Part model, mm, in its own coordinate system. Face numbers are marked on the shaded views. A direction names the side the tool comes from. Round coordinates to 2 decimals unless told otherwise and drop trailing zeros. Order: outer loops, then holes, each group sorted by start corner. A loop starts at its lowest first (then second) coordinate and runs counter-clockwise, first axis right, second up. Notation, with made-up numbers: M 17.5,37 L 33.5,37 A16 ccw 33.5,42 Z; hole C 76.25,-1.75 d3. An arc over 180 degrees is marked long. One line per question, with ' | ' between items.
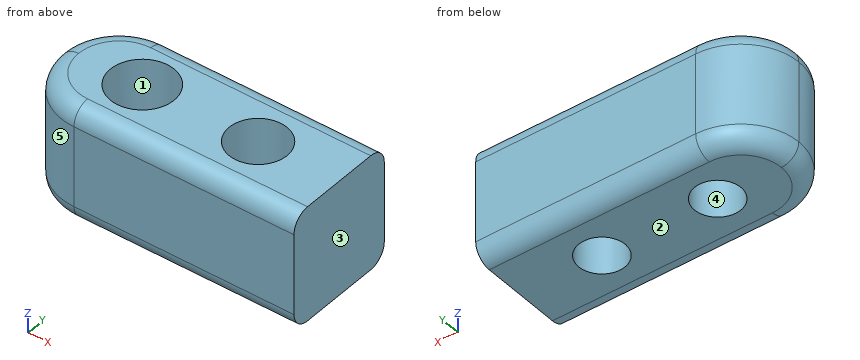
Autodesk Inventor part; units mm, degrees
ref_plane "YZ Plane" through (0, 0, 0) normal (1, 0, 0) x (0, 1, 0)
ref_plane "XZ Plane" through (0, 0, 0) normal (0, 1, 0) x (-1, 0, 0)
ref_plane "XY Plane" through (0, 0, 0) normal (0, 0, 1) x (1, 0, 0)
sketch "Sketch8" plane through (0, 0, 0) normal (0, 0, 1) x (1, 0, 0)
  line L0 (0, 0) -> (-10, 0)
  line L1 (-10, 0) -> (-10, 10)
  line L2 (-10, 10) -> (0, 10)
  line L3 (0, 10) -> (0, 0)
  dimension "d38" = 10
  dimension "d39" = 10
extrude "Extrusion5" add sketch "Sketch8" along normal blind 10
sketch "Sketch9" plane through (0, 0, 10) normal (0, 0, 1) x (1, 0, 0)
  point P0 (0, 0)
  point P1 (-5, 5)
hole "Hole3" at (-5, 5, 10) direction (0, 0, -1) diameter 4 depth 10 counterbore diameter 5.5 counterbore depth 5
sketch "Sketch14" plane through (-10, 0, 0) normal (-1, 0, 0) x (0, 0, 1)
  line L0 (0, 0) -> (10, 0)
  line L1 (10, 0) -> (10, 10)
  line L2 (10, 10) -> (0, 10)
  line L3 (0, 10) -> (0, 0)
  dimension "d71" = 10
  dimension "d72" = 10
extrude "Extrusion9" add sketch "Sketch14" along normal blind 2
fillet "Fillet1" radius 5 2 edges at (-12, 10, 5) (-12, 0, 5)
sketch "Sketch15" plane through (0, 0, 0) normal (1, 0, 0) x (0, 0, -1)
  line L0 (-10, 0) -> (-10, 10)
  line L1 (0, 0) -> (-10, 0)
  line L2 (-10, 0) -> (-10, 10)
  line L3 (-10, 10) -> (0, 10)
  line L4 (0, 10) -> (0, 0)
  dimension "d76" = 10
  dimension "d77" = 10
extrude "Extrusion10" add sketch "Sketch15" along normal blind 10
sketch "Sketch16" plane through (0, 0, 10) normal (0, 0, 1) x (1, 0, 0)
  point P0 (0, 0)
  point P1 (5, 5)
hole "Hole5" at (5, 5, 10) direction (0, 0, -1) diameter 4 depth 10 counterbore diameter 5 counterbore depth 4.5
sketch "Sketch17" plane through (10, 0, 0) normal (1, 0, 0) x (0, 0, -1)
  line L0 (0, 0) -> (-10, 0)
  line L1 (-10, 0) -> (-10, 10)
  line L2 (-10, 10) -> (0, 10)
  line L3 (0, 10) -> (0, 0)
  dimension "d87" = 10
  dimension "d88" = 10
extrude "Extrusion11" add sketch "Sketch17" along normal blind 2
fillet "Fillet2" radius 1.5 6 edges at (-10.5357, 8.5357, 10) (2.4997, 0, 10) (2.4998, 10, 10) (-10.5357, 8.5357, 0) (2.4997, 0, 0) (2.4998, 10, 0)
properties part number "Hole_TestFits"
1) Saw through at C-C (x = 8). List the corners of the cut face in (y, z).
The answers:
outline: M 0,1.5 A1.5 ccw 1.5,0 L 8.5,0 A1.5 ccw 10,1.5 L 10,8.5 A1.5 ccw 8.5,10 L 1.5,10 A1.5 ccw 0,8.5 Z
2) Saw through at A-A (x = 5). List the corners of the cut face in (y, z), plus the area to 3 significant figures.
The answers:
outline: M 0,1.5 A1.5 ccw 1.5,0 L 3,0 L 3,5.5 L 2.5,5.5 L 2.5,10 L 1.5,10 A1.5 ccw 0,8.5 Z; M 7,0 L 8.5,0 A1.5 ccw 10,1.5 L 10,8.5 A1.5 ccw 8.5,10 L 7.5,10 L 7.5,5.5 L 7,5.5 Z | area: 53.6 mm²
3) Two-plate mould, pull along Y, no slides. Class the marked faces 3, 4 and 5: released by +Y, released by -Y, zero draft, split by the parting line, or undercut.
The answers:
face 3: zero draft | face 4: undercut | face 5: released by -Y
4) Probe line 1 (X direction, y = 5, z = 8.5); line 2 (X direction, y = 5, z = 3); line 3 (Y direction, x = 5, z = 2.3). List the from-to ranges inside material, lowest first. Write a range as [from, to].
The answers:
line 1: x = [-12, -7.75], [-2.25, 2.5], [7.5, 12] | line 2: x = [-12, -7], [-3, 3], [7, 12] | line 3: y = [0, 3], [7, 10]
5) Saw through at B-B (z = 4.5). Give the number of separate pieces and of enclosed holes in the cut face, plus the area to 3 significant figures.
The answers:
separate pieces: 1 | enclosed holes: 2 | area: 204 mm²
6) Drop flat-ended pins along their axis: pin 1 (4.5 mm diameter, centred on x = -5, y = 5, fed in from +Z); pin 2 (2 mm diameter, centred on x = -8.5, z = 4.5, fed in from +Y) (3 decimals); pin 3 (3 mm diameter, centred on x = 5, y = 5, fed in from -Z). Give the stop position or say it passes through.
The answers:
pin 1: stops at z = 5 | pin 2: stops at y = 9.975 | pin 3: passes through
7) Which spindle directions (+Z, -Z, +X, -X, +Y, -Y) get a long thin tool onto all of the face, cutting with end or side? Do the marked faces 1 and 2. Say none if no direction does.
The answers:
face 1: +Z | face 2: -Z, +X, -X, +Y, -Y
